The figure shows three views and two pictorial views of one solid part (mm, origin at its lowest corner). Answer the questions. Give positions to 0.01 mm unless a question says otherwise; leave off trailing zeros. Write each loop counter-clockwise with the first axis right and the second up, starting at its lowest first coordinate (ties: lowest second). Pieces come first, ordered by that corner, then holes. Notation, with made-up numbers: (9.25, -33.75) -> (60.25, -33.75) arc R17 cw to (60.25, -5.75) -> close; hole circle Ø1 at (10.5, 82). An arc over 180 degrees is marked (long way). Answer as CSV lines item,"result". Start each with the question number.
1. The part is cut by section A-A, the plane x = 82. Determine the outline of the cut face in (y, z).
2. Find the intervals of material crossed by line 1 (X direction, y = 2.25, z = 2.5); line 2 (X direction, y = 7.25, z = 0.75); line 3 (Z direction, x = 87.5, y = 5.25), in increasing order.
3. Given pin 1 (1.5 mm diameter, centred on x = 16, y = 3, fed in from +Z); pin 2 (2 mm diameter, centred on x = 28.5, z = 9, fed in from +Y), each flat-ended and moving along its own axis, determine where each tip first touches the part or whether it passes through.
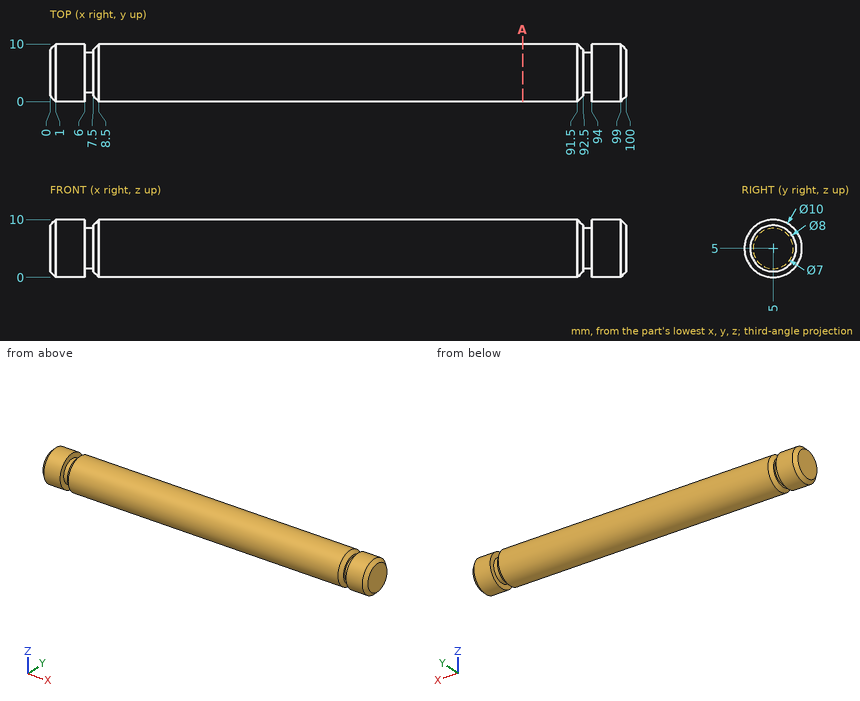
Results found:
1,outline,"circle Ø10 at (5, 5)"
2,line 1,"x = 0 to 6, 7.5 to 92.5, 94 to 100"
2,line 2,"x = 0.81 to 6, 8.31 to 91.69, 94 to 99.19"
2,line 3,"z = 0.01 to 9.99"
3,pin 1,"stops at z = 9.84"
3,pin 2,"stops at y = 9"
